For this review, take the finished solid that the model builds, in its own axes (mm). A direction names the side the tool comes from. Coordinates: 2 decimals unless noted, no trailing zeros. Order: outer loops, then holes, each group sorted by start corner. A loop starts at its lowest first (then second) coordinate and runs counter-clockwise, first axis right, second up. Notation, with made-up numbers: (67, 4) -> (82, 4) arc R17 cw to (82, 23) -> close; hole circle Ø2 at (-27.5, -36.75). An arc over 180 degrees is marked (long way). Write item = value, one per line. Start each with the question number.
1) Draft analysis for pull direction X (two halves, no side actions). For faces 4 (the face through (10, 24, -4)), 5 (the face through (-12.5, 17.5, 0)), 6 (the face through (-11.5, 8, 0)), state which applies: +X half, -X half, draft (parallel to the pull), parting line (faces both ways), or undercut.
2) Machinability: for faces 1 (the face through (8.385, 28.479, -0.751)), 2 (the face through (-15, 18, -0.75)), 3 (the face through (11.5, 21, 0)), which of the approach directions +Z, -Z, +X, -X, +Y, -Y give a long, thin tool a straight path to every point of the face, cutting with its end or side? Answer none if there is none.
3) Consider section B-B on z = 3.25. Give the boundary of the cut face in (x, y), and give its area (3 significant figures).
4) Consider section A-A on x = 0.5. Give the boundary of the cut face in (y, z).
5) Consider section D-D on z = 5. Give the boundary of the cut face in (x, y).
6) Consider section C-C on y = 18.5. Give the boundary of the cut face in (x, z).
7) Wall thickness on probe 1 along Z at (x, y) = (-13.75, 17.2); probe 2 along X at (y, z) = (21.25, -4.5); probe 3 along X at (y, z) = (18.25, 0): over which ranges is each line inside the solid? List them lowest first. Write a range as [from, to].
8) Insertion check: pin 1 Ø2 at (y, z) = (6.5, -3) entering from +X; pin 2 Ø5 at (x, z) = (13.5, 1) entering from +Y; pin 3 Ø5 at (y, z) = (4, 4.5) entering from -X. Each pin has a flat end and moves straight along its axis. Give the tip position at first contact, or say it passes through.
from build123d import *

# Parameters (mm, degrees)
SKETCH1_W                = 23
SKETCH1_H                = 11
BOSS_EXTRUDE1_DEPTH      = 24
SKETCH2_W                = 11
SKETCH2_H                = 3
BOSS_EXTRUDE2_DEPTH      = 4.5
BOSS_EXTRUDE2_DEPTH_BACK = 27.5
SKETCH3_R                = 2.5
BOSS_EXTRUDE3_DEPTH      = 3
SKETCH4_R                = 2.5
BOSS_EXTRUDE4_DEPTH      = 3
BOSS_EXTRUDE4_DEPTH_BACK = 27
CUT_EXTRUDE1_DEPTH       = 4


with BuildPart() as part:
    # Sketch1 → Boss-Extrude1 (new body)
    with BuildSketch(Plane(origin=(0, 0, 0), x_dir=(1, 0, 0), z_dir=(0, 1, 0))):
        Rectangle(SKETCH1_W, SKETCH1_H)
    extrude(amount=BOSS_EXTRUDE1_DEPTH)

    # Sketch2 → Boss-Extrude2 (add, two sides)
    with BuildSketch(Plane(origin=(11.5, 0, 0), x_dir=(0, 0, -1), z_dir=(1, 0, 0))) as boss_extrude2_sk:
        with Locations((0, 17.5)):
            Rectangle(SKETCH2_W, SKETCH2_H)
    extrude(amount=BOSS_EXTRUDE2_DEPTH)
    extrude(boss_extrude2_sk.sketch, amount=-BOSS_EXTRUDE2_DEPTH_BACK)

    # Sketch3 → Boss-Extrude3 (add)
    with BuildSketch(Plane(origin=(0, 24, 0), x_dir=(1, 0, 0), z_dir=(0, 1, 0))):
        with BuildLine():
            Line((-0.5, 2), (0.876524617, 2))
            ThreePointArc((0.876524617, 2), (11.5, 0), (0.876524617, -2))
            Line((0.876524617, -2), (-0.5, -2))
            ThreePointArc((-0.5, -2), (-2.5, 0), (-0.5, 2))
        make_face()
        with Locations((6, 0)):
            Circle(SKETCH3_R, mode=Mode.SUBTRACT)
    extrude(amount=BOSS_EXTRUDE3_DEPTH)

    # Sketch4 → Boss-Extrude4 (add, two sides)
    with BuildSketch(Plane(origin=(0, 27, 0), x_dir=(1, 0, 0), z_dir=(0, 1, 0))) as boss_extrude4_sk:
        with Locations((6, 0)):
            Circle(SKETCH4_R)
    extrude(amount=BOSS_EXTRUDE4_DEPTH)
    extrude(boss_extrude4_sk.sketch, amount=-BOSS_EXTRUDE4_DEPTH_BACK)

    # Sketch5 → Cut-Extrude1 (cut)
    with BuildSketch(Plane(origin=(0, 19, 0), x_dir=(1, 0, 0), z_dir=(0, 1, 0))):
        with BuildLine():
            Line((-16, -0.75), (-14.75, -0.75))
            ThreePointArc((-14.75, -0.75), (-12.5, 0), (-14.75, 0.75))
            Line((-14.75, 0.75), (-16, 0.75))
            Line((-16, 0.75), (-16, -0.75))
        make_face()
        with BuildLine():
            Line((14.75, 0.75), (16, 0.75))
            Line((16, 0.75), (16, -0.75))
            Line((16, -0.75), (14.75, -0.75))
            ThreePointArc((14.75, -0.75), (12.5, 0), (14.75, 0.75))
        make_face()
    extrude(amount=-CUT_EXTRUDE1_DEPTH, mode=Mode.SUBTRACT)


solid = part.part
Answer sheet:
q1.face_4 = draft
q1.face_5 = undercut
q1.face_6 = -X half
q2.face_1 = +Y
q2.face_2 = -X, +Y, -Y
q2.face_3 = +Z, -Z, +X, +Y
q3.outline = (-16, 16) -> (-11.5, 16) -> (-11.5, 0) -> (11.5, 0) -> (11.5, 16) -> (16, 16) -> (16, 19) -> (11.5, 19) -> (11.5, 24) -> (10.44, 24) -> (10.44, 27) -> (1.56, 27) -> (1.56, 24) -> (-11.5, 24) -> (-11.5, 19) -> (-16, 19) -> close
q3.area = 606 mm2
q4.outline = (0, -5.5) -> (24, -5.5) -> (24, -2) -> (27, -2) -> (27, 2) -> (24, 2) -> (24, 5.5) -> (0, 5.5) -> close
q5.outline = (-16, 16) -> (-11.5, 16) -> (-11.5, 0) -> (11.5, 0) -> (11.5, 16) -> (16, 16) -> (16, 19) -> (11.5, 19) -> (11.5, 24) -> (8.29, 24) -> (8.29, 27) -> (3.71, 27) -> (3.71, 24) -> (-11.5, 24) -> (-11.5, 19) -> (-16, 19) -> close
q6.outline = (-16, -5.5) -> (16, -5.5) -> (16, -0.75) -> (14.75, -0.75) arc R1.25 cw (long way) to (14.75, 0.75) -> (16, 0.75) -> (16, 5.5) -> (-16, 5.5) -> (-16, 0.75) -> (-14.75, 0.75) arc R1.25 cw (long way) to (-14.75, -0.75) -> (-16, -0.75) -> close
q7.probe_1 = [-5.5, -1.25], [1.25, 5.5]
q7.probe_2 = [-11.5, 11.5]
q7.probe_3 = [-12.5, 12.5]
q8.pin_1 = 11.5
q8.pin_2 = 27
q8.pin_3 = -11.5
